```python
from build123d import *

# Parameters (mm, degrees)
BOSS_EXTRU_3_DEPTH      = 4
ESQUISSE3_W             = 12
ESQUISSE3_H             = 7
BOSS_EXTRU_4_DEPTH      = 8.5
ENL_V_MAT_EXTRU_1_REACH = 9
ESQUISSE4_R             = 1.65
ESQUISSE4_R_2           = 2.9
ESQUISSE5_R             = 4.1
ENL_V_MAT_EXTRU_2_DEPTH = 6
CONG_1_R                = 4
CONG_2_R                = 2
ESQUISSE6_R             = 3
ENL_V_MAT_EXTRU_3_DEPTH = 3.7
ENL_V_MAT_EXTRU_4_DEPTH = 2


with BuildPart() as part:
    # Esquisse2 → Boss.-Extru.3 (new body)
    with BuildSketch(Plane(origin=(0, 0, 0), x_dir=(1, 0, 0), z_dir=(0, 1, 0))):
        with BuildLine():
            Line((11.568725398, 38.128215269), (18.568725398, 38.128215269))
            ThreePointArc((18.568725398, 38.128215269), (19.275832179, 37.83532205), (19.568725398, 37.128215269))
            Line((19.568725398, 37.128215269), (19.568725398, 35.628215269))
            Line((19.568725398, 35.628215269), (17.068725398, 35.628215269))
            Line((17.068725398, 35.628215269), (17.068725398, 33.128215269))
            Line((17.068725398, 33.128215269), (21.068725398, 33.128215269))
            Line((21.068725398, 33.128215269), (21.068725398, 26.128215269))
            Line((21.068725398, 26.128215269), (9.068725398, 26.128215269))
            Line((9.068725398, 26.128215269), (9.068725398, 33.128215269))
            Line((9.068725398, 33.128215269), (13.068725398, 33.128215269))
            Line((13.068725398, 33.128215269), (13.068725398, 35.628215269))
            Line((13.068725398, 35.628215269), (10.568725398, 35.628215269))
            Line((10.568725398, 35.628215269), (10.568725398, 37.128215269))
            ThreePointArc((10.568725398, 37.128215269), (10.861618616, 37.83532205), (11.568725398, 38.128215269))
        make_face()
    extrude(amount=BOSS_EXTRU_3_DEPTH)

    # Esquisse3 → Boss.-Extru.4 (add)
    with BuildSketch(Plane(origin=(0, 4, 0), x_dir=(1, 0, 0), z_dir=(0, 1, 0))):
        with Locations((15.068725398, 29.628215269)):
            Rectangle(ESQUISSE3_W, ESQUISSE3_H)
    extrude(amount=BOSS_EXTRU_4_DEPTH)

    # Symétrie1: part across plane


with BuildPart() as part_1:
    add(part.part)
    add(part.part.mirror(Plane.ZX.offset(12.5)))

    # Esquisse4 → Enlèv. mat.-Extru.1 (cut, up to next)
    with BuildSketch(Plane(origin=(0, 0, -33.128215269), x_dir=(-1, 0, 0), z_dir=(0, 0, -1)), mode=Mode.PRIVATE) as enl_v_mat_extru_1_sk1:
        with Locations((-15.068725398, 8)):
            Circle(ESQUISSE4_R)
    enl_v_mat_extru_1_tool1 = extrude(enl_v_mat_extru_1_sk1.sketch, amount=-ENL_V_MAT_EXTRU_1_REACH, mode=Mode.PRIVATE) & part_1.part
    add(enl_v_mat_extru_1_tool1.solids().sort_by_distance((15.068725, 8, -33.128215))[0], mode=Mode.SUBTRACT)
    # Esquisse4 → Enlèv. mat.-Extru.1 (cut, up to next)
    with BuildSketch(Plane(origin=(0, 0, -33.128215269), x_dir=(-1, 0, 0), z_dir=(0, 0, -1)), mode=Mode.PRIVATE) as enl_v_mat_extru_1_sk2:
        with Locations((-15.068725398, 16)):
            Circle(ESQUISSE4_R_2)
    enl_v_mat_extru_1_tool2 = extrude(enl_v_mat_extru_1_sk2.sketch, amount=-ENL_V_MAT_EXTRU_1_REACH, mode=Mode.PRIVATE) & part_1.part
    add(enl_v_mat_extru_1_tool2.solids().sort_by_distance((15.068725, 16, -33.128215))[0], mode=Mode.SUBTRACT)

    # Esquisse5 → Enlèv. mat.-Extru.2 (cut)
    with BuildSketch(Plane(origin=(0, 0, -33.128215269), x_dir=(-1, 0, 0), z_dir=(0, 0, -1))):
        with Locations((-15.068725398, 16)):
            Circle(ESQUISSE5_R)
    extrude(amount=-ENL_V_MAT_EXTRU_2_DEPTH, mode=Mode.SUBTRACT)

    # Congé1
    cong_1_edges = [part_1.edges().sort_by_distance(p)[0] for p in [
        (9.068725398, 0, -29.628215269),
        (9.068725398, 25, -29.628215269),
        (21.068725398, 0, -29.628215269),
        (21.068725398, 25, -29.628215269),
    ]]
    fillet(cong_1_edges, radius=CONG_1_R)

    # Congé2
    cong_2_edges = [part_1.edges().sort_by_distance(p)[0] for p in [
        (9.068725398, 12.5, -26.128215269),
        (15.068725398, 0, -26.128215269),
        (21.068725398, 12.5, -26.128215269),
        (15.068725398, 25, -26.128215269),
        (19.897152522, 23.828427125, -26.128215269),
        (19.897152522, 1.171572875, -26.128215269),
        (10.240298273, 23.828427125, -26.128215269),
        (10.240298273, 1.171572875, -26.128215269),
    ]]
    fillet(cong_2_edges, radius=CONG_2_R)

    # Esquisse6 → Enlèv. mat.-Extru.3 (cut)
    with BuildSketch(Plane.XY.offset(-26.128215269)):
        with Locations((15.068725398, 8)):
            Circle(ESQUISSE6_R)
    extrude(amount=-ENL_V_MAT_EXTRU_3_DEPTH, mode=Mode.SUBTRACT)

    # Esquisse7 → Enlèv. mat.-Extru.4 (cut)
    with BuildSketch(Plane(origin=(0, 0, -33.128215269), x_dir=(-1, 0, 0), z_dir=(0, 0, -1))):
        Polygon((-16.714173665, 10.85), (-13.42327713, 10.85), (-11.777828863, 8), (-13.42327713, 5.15), (-16.714173665, 5.15), (-18.359621932, 8), align=None)
    extrude(amount=-ENL_V_MAT_EXTRU_4_DEPTH, mode=Mode.SUBTRACT)


solid = part_1.part
```
Here's how the part is built. I have some questions about the finished solid (model axes, mm). A direction names the side the tool comes from. Give positions to 0.01 mm unless a question says otherwise; leave off trailing zeros. Order: outer loops, then holes, each group sorted by start corner. A loop starts at its lowest first (then second) coordinate and runs counter-clockwise, first axis right, second up. Notation, with made-up numbers: M -17,24 L 42,24 A15 ccw 42,44 Z; hole C -20,-9 d3. An arc over 180 degrees is marked long. Use a Markdown table: item, result. Add a question column.
1. On a 3-axis mill with a long thin cutter (end or side, diameter ignored), from which of +Z, -Z, +X, -X, +Y, -Y can I reach the whole of each face in a straight line? I mean faces 4 (the cylindrical face through (19.866, 23.859, -30.593)), 5 (the flat face through (17.548, 9.405, -32.142)), 6 (the cylindrical face through (19.866, 1.141, -30.593)), 7 (the cylindrical face through (17.93, 8.9, -27.95)), 8 (the flat face through (13.069, 2, -34)). Say none if no direction works.
2. Suppose I cut it at C-C (z = -34.25). List the corners of the cut face in (x, y) for me.
3. Suppose I cut it at D-D (x = 13.75). Give the number of separate pieces and of enclosed holes in the cut face, and give its area (3 significant figures).
4. Suppose I cut it at A-A (y = 16). List the corners of the cut face in (x, z) for me, and give its area (3 significant figures).
5. I need wall thicknesses on probe 1 along Y at (x, z) = (15.25, -32); probe 2 along Y at (x, z) = (15.25, -29.5); probe 3 along Y at (x, z) = (10.75, -36). Which ranges of each line are inside material? Lowest first, please. Write a range as from..to.
6. For pin 1 Ø0.8 at (y, z) = (2, -36) entering from -X; pin 2 Ø1.2 at (x, y) = (11.5, 1.5) entering from +Z; pin 3 Ø0.8 at (y, z) = (23, -36.5) entering from +X; pin 4 Ø2.5 at (x, y) = (15.5, 17) entering from -Z, each with a flat end and sliding along its axis, tell me the tip position at first contact or that it passes through.
7. If we mould it in two halves opening along X, with no side actions, what happens to faces 1 (the cylindrical face through (10.21, 23.8, -30.66)), 2 (the flat face through (12.59, 6.59, -32.14)), 3 (the flat face through (18, 2, -35.628))? For each: +X half, -X half, draft (parallel to the pull), parting line (faces both ways), or undercut.
8. Suppose I cut it at B-B (z = -29). List the corners of the cut face in (x, y) for me.
Results list:
| question | item | result |
|---|---|---|
| 1 | face 4 | +Z, +X, +Y |
| 1 | face 5 | -Z |
| 1 | face 6 | +Z, +X, -Y |
| 1 | face 7 | +Z |
| 1 | face 8 | -X, +Y, -Y |
| 2 | outline | M 13.07,0 L 17.07,0 L 17.07,4 L 13.07,4 Z; M 13.07,21 L 17.07,21 L 17.07,25 L 13.07,25 Z |
| 3 | separate pieces | 3 |
| 3 | enclosed holes | 0 |
| 3 | area | 128 mm² |
| 4 | outline | M 9.07,-33.13 L 10.97,-33.13 L 10.97,-27.13 L 12.17,-27.13 L 12.17,-26.13 L 11.07,-26.13 A2 ccw 9.07,-28.13 Z; M 17.97,-27.13 L 19.17,-27.13 L 19.17,-33.13 L 21.07,-33.13 L 21.07,-28.13 A2 ccw 19.07,-26.13 L 17.97,-26.13 Z |
| 4 | area | 27.3 mm² |
| 5 | probe 1 | y = 0..5.15, 10.85..11.9, 20.1..25 |
| 5 | probe 2 | y = 0..5.01, 10.99..11.9, 20.1..25 |
| 5 | probe 3 | y = 0..4, 21..25 |
| 6 | pin 1 | stops at x = 10.57 |
| 6 | pin 2 | stops at z = -26.16 |
| 6 | pin 3 | stops at x = 19.57 |
| 6 | pin 4 | passes through |
| 7 | face 1 | -X half |
| 7 | face 2 | undercut |
| 7 | face 3 | draft |
| 8 | outline | M 9.07,4 A4 ccw 13.07,0 L 17.07,0 A4 ccw 21.07,4 L 21.07,21 A4 ccw 17.07,25 L 13.07,25 A4 ccw 9.07,21 Z; hole C 15.07,16 d8.2; hole C 15.07,8 d6 |
